```python
from build123d import *

# Parameters (mm, degrees)
F0_R     = 3
F1_DEPTH = 835


# Not quite as in the source:
# - ends of sketch curves that miss each other by under 0.0002 mm in the source are joined


with BuildPart() as f1:
    # F0 (on Right) → F1 (new body)
    with BuildSketch(Plane.YZ):
        with BuildLine():
            Line((12.5, -11.85), (15, -11.85))
            Line((15, -11.85), (15, 11.85))
            Line((15, 11.85), (12.5, 11.85))
            Line((12.5, 11.85), (12.5, 9.85))
            Line((12.5, 9.85), (6.547707, 9.85))
            ThreePointArc((6.5477069495, 9.8499999523), (4.5, 15), (6.5477069495, 20.1500000477))
            Line((6.547707, 20.15), (12.5, 20.15))
            Line((12.5, 20.15), (12.5, 18.15))
            Line((12.5, 18.15), (15, 18.15))
            Line((15, 18.15), (15, 30))
            Line((15, 30), (3.15, 30))
            Line((3.15, 30), (3.15, 27.5))
            Line((3.15, 27.5), (5.15, 27.5))
            Line((5.15, 27.5), (5.15, 21.547707))
            ThreePointArc((5.1500000477, 21.5477069495), (0, 19.5), (-5.1500000477, 21.5477069495))
            Line((-5.15, 21.547707), (-5.15, 27.5))
            Line((-5.15, 27.5), (-3.15, 27.5))
            Line((-3.15, 27.5), (-3.15, 30))
            Line((-3.15, 30), (-15, 30))
            Line((-15, 30), (-15, 18.15))
            Line((-15, 18.15), (-12.5, 18.15))
            Line((-12.5, 18.15), (-12.5, 20.15))
            Line((-12.5, 20.15), (-6.547707, 20.15))
            ThreePointArc((-6.5477069495, 20.1500000477), (-4.5, 15), (-6.5477069495, 9.8499999523))
            Line((-6.547707, 9.85), (-12.5, 9.85))
            Line((-12.5, 9.85), (-12.5, 11.85))
            Line((-12.5, 11.85), (-15, 11.85))
            Line((-15, 11.85), (-15, -11.85))
            Line((-15, -11.85), (-12.5, -11.85))
            Line((-12.5, -11.85), (-12.5, -9.85))
            Line((-12.5, -9.85), (-6.547707, -9.85))
            ThreePointArc((-6.5477069495, -9.8499999523), (-4.5, -15), (-6.5477069495, -20.1500000477))
            Line((-6.547707, -20.15), (-12.5, -20.15))
            Line((-12.5, -20.15), (-12.5, -18.15))
            Line((-12.5, -18.15), (-15, -18.15))
            Line((-15, -18.15), (-15, -30))
            Line((-15, -30), (-3.15, -30))
            Line((-3.15, -30), (-3.15, -27.5))
            Line((-3.15, -27.5), (-5.15, -27.5))
            Line((-5.15, -27.5), (-5.15, -21.547707))
            ThreePointArc((-5.1500000477, -21.5477069495), (0, -19.5), (5.1500000477, -21.5477069495))
            Line((5.15, -21.547707), (5.15, -27.5))
            Line((5.15, -27.5), (3.15, -27.5))
            Line((3.15, -27.5), (3.15, -30))
            Line((3.15, -30), (15, -30))
            Line((15, -30), (15, -18.15))
            Line((15, -18.15), (12.5, -18.15))
            Line((12.5, -18.15), (12.5, -20.15))
            Line((12.5, -20.15), (6.547707, -20.15))
            ThreePointArc((6.5477069495, -20.1500000477), (4.5, -15), (6.5477069495, -9.8499999523))
            Line((6.547707, -9.85), (12.5, -9.85))
            Line((12.5, -9.85), (12.5, -11.85))
        make_face()
        with Locations((-10, -25)):
            Circle(F0_R, mode=Mode.SUBTRACT)
        with Locations((10, -25)):
            Circle(F0_R, mode=Mode.SUBTRACT)
        with Locations((-10, 25)):
            Circle(F0_R, mode=Mode.SUBTRACT)
        with BuildLine():
            ThreePointArc((-12, 3.85), (-11.1213203436, 5.9713203436), (-9, 6.85))
            Line((-9, 6.85), (-4.705405, 6.85))
            Line((-4.705405, 6.85), (-1.25, 12.834936))
            ThreePointArc((-1.25, 12.834936), (0, 17.5), (1.2499997876, 12.8349363679))
            Line((1.2499997876, 12.8349363679), (4.705405, 6.85))
            Line((4.705405, 6.85), (9, 6.85))
            ThreePointArc((9, 6.85), (11.1213203436, 5.9713203436), (12, 3.85))
            Line((12, 3.85), (12, -3.85))
            ThreePointArc((12, -3.85), (11.1213203436, -5.9713203436), (9, -6.85))
            Line((9, -6.85), (4.705405, -6.85))
            Line((4.705405, -6.85), (1.25, -12.834937))
            ThreePointArc((1.25, -12.834937), (0, -17.5), (-1.2500002206, -12.8349366179))
            Line((-1.2500002206, -12.8349366179), (-4.705405, -6.85))
            Line((-4.705405, -6.85), (-9, -6.85))
            ThreePointArc((-9, -6.85), (-11.1213203436, -5.9713203436), (-12, -3.85))
            Line((-12, -3.85), (-12, 3.85))
        make_face(mode=Mode.SUBTRACT)
        with Locations((10, 25)):
            Circle(F0_R, mode=Mode.SUBTRACT)
    extrude(amount=F1_DEPTH)


solid = f1.part
```
The model under review builds one solid part; all positions refer to its coordinate system, in mm. Coordinates: 2 decimals unless noted, no trailing zeros.
1) To check wall thickness, follow probe 1 along Z at (x, y) = (369.5, -10); probe 2 along Z at (x, y) = (593, 9.5); probe 3 along Z at (x, y) = (798, 0.5). State the ranges of each line that lie inside material, in increasing order.
2) Clearance check with flat-ended pins moving along their axes: pin 1 Ø3.5 at (y, z) = (-10, 25) entering from +X; pin 2 Ø3 at (x, z) = (595, -13.5) entering from -Y. State where each tip first meets the part, or that it passes through.
3) We need section A-A on x = 172. Count the separate pieces of the cut face and the enclosed holes in it, then the cut area to 3 significant figures.
Answer list:
1. probe 1: z = -30 to -28, -22 to -20.15, -9.85 to -6.68, 6.68 to 9.85, 20.15 to 22, 28 to 30
1. probe 2: z = -30 to -27.96, -22.04 to -20.15, -9.85 to -6.81, 6.81 to 9.85, 20.15 to 22.04, 27.96 to 30
1. probe 3: z = -19.52 to -17.45, 17.45 to 19.52
2. pin 1: passes through
2. pin 2: stops at y = -5.13
3. separate pieces: 1
3. enclosed holes: 5
3. area: 707 mm2
